Design review of the part built by this model. Coordinates are the model's own, in mm. A direction names the side the tool comes from. Give positions to 0.01 mm unless a question says otherwise; leave off trailing zeros. Write each loop counter-clockwise with the first axis right and the second up, starting at its lowest first coordinate (ties: lowest second). Pieces come first, ordered by that corner, then holes. Notation, with made-up numbers: (-36.5, 3) -> (15.5, 3) arc R28 cw to (15.5, 28) -> close; hole circle Ø5 at (2, 31). An arc over 180 degrees is marked (long way). Put each result on its own line as item: value. Start each with the question number.
from build123d import *

# Parameters (mm, degrees)
SKETCH1_R           = 2
SKETCH1_W           = 6.4
SKETCH1_H           = 6.4
BOSS_EXTRUDE1_DEPTH = 3
SKETCH1_3_W         = 6.4
SKETCH1_3_H         = 6.4
BOSS_EXTRUDE2_DEPTH = 6


with BuildPart() as part:
    # Sketch1 → Boss-Extrude1 (new body)
    # profile 1 of 2: a face of its own
    with BuildSketch(Plane(origin=(0, 0, 0), x_dir=(0, 0, -1), z_dir=(1, 0, 0))):
        with BuildLine():
            Line((8, 5), (-8, 5))
            ThreePointArc((-8, 5), (-9.414213562, 4.414213562), (-10, 3))
            Line((-10, 3), (-10, -3))
            ThreePointArc((-10, -3), (-9.414213562, -4.414213562), (-8, -5))
            Line((-8, -5), (8, -5))
            ThreePointArc((8, -5), (9.414213562, -4.414213562), (10, -3))
            Line((10, -3), (10, 3))
            ThreePointArc((10, 3), (9.414213562, 4.414213562), (8, 5))
        make_face()
        with Locations((-5, 0)):
            Circle(SKETCH1_R, mode=Mode.SUBTRACT)
        with Locations((5, 0)):
            Rectangle(SKETCH1_W, SKETCH1_H, mode=Mode.SUBTRACT)
    # profile 2 of 2: a face of its own
    with BuildSketch(Plane(origin=(0, 0, 0), x_dir=(0, 0, -1), z_dir=(1, 0, 0))):
        with Locations((5, 0)):
            Rectangle(SKETCH1_W, SKETCH1_H)
    extrude(amount=BOSS_EXTRUDE1_DEPTH)

    # Sketch1_3 → Boss-Extrude2 (add)
    with BuildSketch(Plane(origin=(0, 0, 0), x_dir=(0, 0, -1), z_dir=(1, 0, 0))):
        with Locations((5, 0)):
            Rectangle(SKETCH1_3_W, SKETCH1_3_H)
    extrude(amount=BOSS_EXTRUDE2_DEPTH)


solid = part.part
Q1. For pin 1 (1.5 mm diameter, centred on y = -3, z = 1, fed in from +X); pin 2 (1.5 mm diameter, centred on x = 4, z = -3.5, fed in from -Y), all flat-tipped, find the tip position at first contact; note any pin that passes through.
Q2. Mouldability with a two-part tool opening along Y and no side actions: class faces 6 (the face through (4, 3.2, -5)), 7 (the face through (0, 0, 0)), 8 (the face through (1.5, -1.2, 6.6)) as +Y half, -Y half, draft (parallel to the pull), parting line (faces both ways), or undercut.
Q3. To check wall thickness, follow probe 1 along Y at (x, z) = (1.3, 5); probe 2 along X at (y, z) = (4.25, -2); probe 3 along Y at (x, z) = (4.8, -2.25). State the ranges of each line that lie inside material, in increasing order. Write a range as from..to.
Q4. Take a section at C-C on z = -7.75. Give the boundary of the cut face in (x, y), then the cut area to 3 significant figures.
Q5. Take a section at D-D on z = 5. Give the boundary of the cut face in (x, y).
Q6. Take a section at A-A on y = 0. Give the boundary of the cut face in (x, z), then the cut area to 3 significant figures.
Q7. Take a section at B-B on x = 1.8. Give the boundary of the cut face in (y, z), then the cut area to 3 significant figures.
Q8. Machinability: for faces 1 (the face through (1, 0, 10)), 2 (the face through (4, -3.2, -5)), 3 (the face through (4, 0, -8.2)), 4 (the face through (1, 0, -10)), 5 (the face through (4, 0, -1.8)), which of the approach directions +Z, -Z, +X, -X, +Y, -Y give a long, thin tool a straight path to every point of the face, cutting with its end or side? Answer none if there is none.
Result:
1. pin 1: stops at x = 3
1. pin 2: stops at y = -3.2
2. face 6: +Y half
2. face 7: draft
2. face 8: undercut
3. probe 1: y = -5..-2, 2..5
3. probe 2: x = 0..3
3. probe 3: y = -3.2..3.2
4. outline: (0, -5) -> (3, -5) -> (3, -3.2) -> (6, -3.2) -> (6, 3.2) -> (3, 3.2) -> (3, 5) -> (0, 5) -> close
4. area: 49.2 mm^2
5. outline: (0, -5) -> (3, -5) -> (3, -2) -> (0, -2) -> close; (0, 2) -> (3, 2) -> (3, 5) -> (0, 5) -> close
6. outline: (0, -10) -> (3, -10) -> (3, -8.2) -> (6, -8.2) -> (6, -1.8) -> (3, -1.8) -> (3, 3) -> (0, 3) -> close; (0, 7) -> (3, 7) -> (3, 10) -> (0, 10) -> close
6. area: 67.2 mm^2
7. outline: (-5, -8) arc R2 ccw to (-3, -10) -> (3, -10) arc R2 ccw to (5, -8) -> (5, 8) arc R2 ccw to (3, 10) -> (-3, 10) arc R2 ccw to (-5, 8) -> close; hole circle Ø4 at (0, 5)
7. area: 184 mm^2
8. face 1: +Z, +X, -X, +Y, -Y
8. face 2: +Z, -Z, +X, -Y
8. face 3: -Z, +X, +Y, -Y
8. face 4: -Z, +X, -X, +Y, -Y
8. face 5: +Z, +X, +Y, -Y
